Read the model definition and answer for the solid it produces. Units are mm, in the model's axes. A direction names the side the tool comes from. Coordinates: 2 decimals unless noted, no trailing zeros. Write each loop counter-clockwise with the first axis right and the second up, starting at its lowest first coordinate (ties: lowest second). Pieces come first, ordered by that corner, then holes.
(1) The part is cut by section A-A, the plane x = 40. State how many separate pieces and enclosed holes the cut face has, and give its area (3 significant figures).
(2) The part is cut by section B-B, the plane z = -18. Determine the outline of the cut face in (x, y).
(3) Given pin 1 (8 mm diameter, centred on x = 11, z = -27, fed in from -Y); pin 2 (12 mm diameter, centred on x = -15, y = -34.5, fed in from +Z); pin 3 (7.5 mm diameter, centred on x = -40.5, y = 0.5, fed in from +Z), each flat-ended and moving along its own axis, determine where each tip first touches the part or whether it passes through.
(4) The part is cut by section C-C, the plane z = 60. Determine the outline of the cut face in (x, y), and give its area (3 significant figures).
(5) Determine the mould class of faces 5 (the flat face through (-12.012, -36, 48)), 6 (the cylindrical face through (39.563, -0.25, 19.613)), 7 (the flat face through (3.33, -44.45, 46.47)) for opening direction Y: pulls with the +Y half, pulls with the -Y half, needs draft (parallel to the pull), parting line crosses it, or undercut.
(6) Which of the six approach directions +Z, -Z, +X, -X, +Y, -Y give full straight-line access (tool end or side, diameter ignored) to faces 1 (the flat face through (40, -8.73, 4)), 2 (the cylindrical face through (-0.688, -53.842, 43.267)), 3 (the flat face through (-33, -20, 38.746)), 4 (the flat face through (-12.929, -45, -49))?
(7) The part is cut by section D-D, the plane z = -42.5. Determine the outline of the cut face in (x, y).
(8) Straight lines are drawn through the part: line 1 along Y through (x, z) = (0, 0); line 2 along Y through (x, z) = (0, -28.5); line 3 along X through (y, z) = (0, -26). For each, find the intervals that lie inside material, in ascending order.
```python
from build123d import *

# Parameters (mm, degrees)
F3_DEPTH       = 87.884
F4_R           = 37.6973348858
F5_DEPTH       = 98.044
F7_DEPTH       = 44.45
F8_R           = 3.175
F9_DEPTH       = 19.05
F11_DEPTH      = 67.564
F11_DEPTH_BACK = 62.992


with BuildPart() as f1:
    # F0 (on Front) → F1 (revolve)
    with BuildSketch(Plane.XZ):
        Polygon((0, 38.7462731748), (-38.1, 38.7462731748), (-57.15, -61.0518104742), (0, -61.0518104742), align=None)
        Polygon((-44.45, 38.7462731748), (-38.1, 38.7462731748), (0, 38.7462731748), (0, 77.8838843107), align=None)
    revolve(axis=Axis((0, 0, -11.1527686497), (0, 0, 1)))

    # F2 (on Front) → F3 (cut)
    with BuildSketch(Plane.XZ):
        Polygon((12.4711716, -36.5671299331), (0, -36.5671299331), (-12.9288284, -36.5671299331), (-12.9288284, -61.0518104742), (0, -61.0518104742), (12.4711716, -61.0518104742), align=None)
    extrude(amount=F3_DEPTH, mode=Mode.SUBTRACT)

    # F4 (on face) → F5 (cut)
    with BuildSketch(Plane(origin=(0, 0, -61.0518104742), x_dir=(1, 0, 0), z_dir=(0, 0, -1))):
        Circle(F4_R)
    extrude(amount=-F5_DEPTH, mode=Mode.SUBTRACT)

    # F6 (on Front) → F7 (join)
    with BuildSketch(Plane.XZ):
        Polygon((-12.0120554089, 38.7462731748), (0, 38.7462731748), (13.3879445911, 38.7462731748), (13.3879445911, 53.9862731748), (0, 53.9862731748), (-12.0120554089, 53.9862731748), align=None)
    extrude(amount=F7_DEPTH)

    # F8 (on face) → F9 (join)
    with BuildSketch(Plane.XZ.offset(44.45)):
        with Locations((0, 46.3662731748)):
            Circle(F8_R)
    extrude(amount=F9_DEPTH)

    # F10 (on Right) → F11 (cut, two sides)
    with BuildSketch(Plane.YZ) as f11_sk:
        with BuildLine():
            ThreePointArc((8.1476010382, 11.462922208), (-0.4339928104, 19.6117778709), (-8.7295742705, 11.1719360575))
            Line((-8.7295742705, 11.1719360575), (-8.7295742705, -3.6683375947))
            Line((-8.7295742705, -3.6683375947), (8.1476010382, -3.6683375947))
            Line((8.1476010382, -3.6683375947), (8.1476010382, 11.462922208))
        make_face()
    extrude(amount=-F11_DEPTH, mode=Mode.SUBTRACT)
    extrude(f11_sk.sketch, amount=F11_DEPTH_BACK, mode=Mode.SUBTRACT)


solid = f1.part
```
Computed:
1. separate pieces: 2
1. enclosed holes: 1
1. area: 4,450 mm2
2. outline: circle Ø97.86 at (0, 0); hole circle Ø75.39 at (0, 0)
3. pin 1: stops at y = -50.54
3. pin 2: stops at z = 53.99
3. pin 3: stops at z = 45.52
4. outline: circle Ø40.62 at (0, 0)
4. area: 1,300 mm2
5. face 5: needs draft
5. face 6: undercut
5. face 7: pulls with the -Y half
6. face 1: +X, -X
6. face 2: -Y
6. face 3: none
6. face 4: -Z, -Y
7. outline: (-12.93, -52.03) - (-12.93, -35.41) arc R37.7 cw (long way) to (12.47, -35.57) - (12.47, -52.14) arc R53.61 ccw (long way) to start
8. line 1: y = -45.5 to -37.7, 37.7 to 45.5
8. line 2: y = -50.94 to -37.7, 37.7 to 50.94
8. line 3: x = -50.46 to -37.7, 37.7 to 50.46
